```python
from build123d import *

# Parameters (mm, degrees)
SKETCH1_W           = 20
SKETCH1_H           = 20
BOSS_EXTRUDE1_DEPTH = 3
SKETCH2_W           = 10
SKETCH2_H           = 1.5
CUT_EXTRUDE1_DEPTH  = 21
SKETCH3_W           = 10
SKETCH3_H           = 1.5
CUT_EXTRUDE2_DEPTH  = 21


with BuildPart() as part:
    # Sketch1 → Boss-Extrude1 (new body)
    with BuildSketch(Plane(origin=(0, 0, 0), x_dir=(1, 0, 0), z_dir=(0, 1, 0))):
        Rectangle(SKETCH1_W, SKETCH1_H)
        Polygon((-8, 1), (-3, 1), (-3, -8), (3, -8), (3, 1), (8, 1), (0, 8), align=None, mode=Mode.SUBTRACT)
    extrude(amount=BOSS_EXTRUDE1_DEPTH)

    # Sketch2 → Cut-Extrude1 (cut, through all)
    with BuildSketch(Plane.XY.offset(10)):
        with Locations((0, 1.5)):
            Rectangle(SKETCH2_W, SKETCH2_H)
    extrude(amount=-CUT_EXTRUDE1_DEPTH, mode=Mode.SUBTRACT)

    # Sketch3 → Cut-Extrude2 (cut, through all)
    with BuildSketch(Plane(origin=(10, 0, 0), x_dir=(0, 0, -1), z_dir=(1, 0, 0))):
        with Locations((0, 1.5)):
            Rectangle(SKETCH3_W, SKETCH3_H)
    extrude(amount=-CUT_EXTRUDE2_DEPTH, mode=Mode.SUBTRACT)


solid = part.part
```
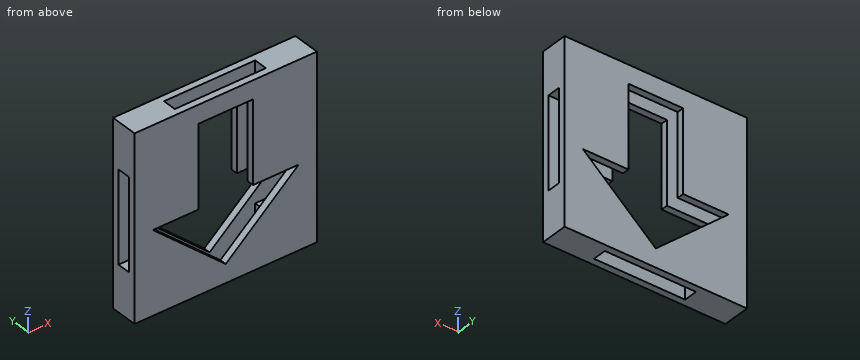
Input: part model. Units: mm. Frame: model coordinates. Round coordinates to 2 decimals unless told otherwise and drop trailing zeros. Order: outer loops, then holes, each group sorted by start corner. A loop starts at its lowest first (then second) coordinate and runs counter-clockwise, first axis right, second up. Notation, with made-up numbers: (8, 6.25) - (16, 6.25) arc R7 cw to (16, 11.25) - close; hole circle Ø8 at (86.5, 22). An arc over 180 degrees is marked (long way). Answer in a Markdown table with one row per item.
Item 1: Section query C-C (x = -8.25). Return the cut outline in (y, z), then the cut area to 3 significant figures.
Model answer:
| item | result |
|---|---|
| outline | (0, -10) - (3, -10) - (3, 10) - (0, 10) - close; hole (0.75, -5) - (2.25, -5) - (2.25, 5) - (0.75, 5) - close |
| area | 45.0 mm² |
Item 2: Line query: line 1 (Y direction, x = 8.75, z = -2.25); line 2 (X direction, y = 2.15, z = -8.75); line 3 (X direction, y = 0.4, z = 6.25). Output: solid intervals per line, ascending.
Model answer:
| item | result |
|---|---|
| line 1 | y = 0 to 0.75, 2.25 to 3 |
| line 2 | x = -10 to -5, 5 to 10 |
| line 3 | x = -10 to -3, 3 to 10 |
Item 3: Section query D-D (z = 7.5). Return the cut outline in (x, y), then the cut area to 3 significant figures.
Model answer:
| item | result |
|---|---|
| outline | (-10, 0) - (-3, 0) - (-3, 0.75) - (-5, 0.75) - (-5, 2.25) - (-3, 2.25) - (-3, 3) - (-10, 3) - close; (3, 0) - (10, 0) - (10, 3) - (3, 3) - (3, 2.25) - (5, 2.25) - (5, 0.75) - (3, 0.75) - close |
| area | 36.0 mm² |
Item 4: Section query A-A (y = 1.1). Return the cut outline in (x, z).
Model answer:
| item | result |
|---|---|
| outline | (-10, -10) - (-5, -10) - (-5, -5) - (-10, -5) - close; (-10, 5) - (-5, 5) - (-5, 10) - (-10, 10) - close; (5, -10) - (10, -10) - (10, -5) - (5, -5) - close; (5, 5) - (10, 5) - (10, 10) - (5, 10) - close |
Item 5: Section query B-B (z = 0). Return the cut outline in (x, y).
Model answer:
| item | result |
|---|---|
| outline | (-10, 0) - (-3, 0) - (-3, 0.75) - (-10, 0.75) - close; (-10, 2.25) - (-3, 2.25) - (-3, 3) - (-10, 3) - close; (3, 0) - (10, 0) - (10, 0.75) - (3, 0.75) - close; (3, 2.25) - (10, 2.25) - (10, 3) - (3, 3) - close |
